Part model, mm, in its own coordinate system. Face numbers are marked on the shaded views. Round coordinates to 2 decimals unless told otherwise and drop trailing zeros. Loops run counter-clockwise (first coordinate to the right, second up) from the corner with the lowest first, then second, coordinate; pieces in that order, holes last.
1) Band-saw the part on D-D, the plane y = -23. Write the cut outline in (x, z), then the cut area to 3 significant figures.
2) Probe line 1 (Z direction, x = 17.5, y = 16); line 2 (Z direction, x = 5.5, y = 19.5); line 3 (Z direction, x = 2.5, y = 2). List the from-to ranges inside material, lowest first.
3) Band-saw the part on A-A, the plane y = 0. Write the cut outline in (x, z), then the cut area to 3 significant figures.
4) Band-saw the part on C-C, the plane x = -23. Write the cut outline in (y, z).
5) Band-saw the part on B-B, the plane z = 61.5. Write the cut outline in (x, y).
6) Drop flat-ended pins along their axis: P1, Ø8, axis at x = -9.5, y = 5, coming from the -Z side; P2, Ø9.5, axis at y = 38.5, z = -6.5, coming from the +X side; P3, Ø10, axis at y = -19, z = 82.5, coming from the +X side; P4, Ø7, axis at y = 26.5, z = -8.5, coming from the -X side. Give the stop position or say it passes through.
7) Mould opens along Z. For the marked faces 1, 2 and 3 say: +Z half, -Z half, draft (parallel to the pull), parting line (faces both ways), or undercut.
from build123d import *

# Parameters (mm, degrees)
SKETCH1_R                = 13.7
BOSS_EXTRUDE1_DEPTH      = 101
SKETCH5_W                = 55.5
SKETCH5_H                = 56.561345004
BOSS_EXTRUDE2_DEPTH      = 2.6
CUT_EXTRUDE4_DEPTH       = 2.6
BOSS_EXTRUDE4_DEPTH      = 6
SKETCH8_W                = 33.3
SKETCH8_H                = 11.7
BOSS_EXTRUDE5_DEPTH      = 2.8
SKETCH9_W                = 33.3
SKETCH9_H                = 2.7
BOSS_EXTRUDE6_DEPTH      = 22.2
FILLET2_R                = 5
REVOLVE1_ANGLE           = 40
REVOLVE1_OTHER_WAY_ANGLE = 40
FILLET4_R                = 6
FILLET5_R                = 6


with BuildPart() as part:
    # Sketch1 → Boss-Extrude1 (new body)
    with BuildSketch(Plane.XY):
        with Locations(Location((0, 0, 0), (0, 0, 180))):
            Circle(SKETCH1_R)
    extrude(amount=BOSS_EXTRUDE1_DEPTH)

    # Sketch5 → Boss-Extrude2 (add)
    with BuildSketch(Plane(origin=(0, 0, 0), x_dir=(-1, 0, 0), z_dir=(0, 0, -1))):
        Rectangle(SKETCH5_W, SKETCH5_H)
    extrude(amount=BOSS_EXTRUDE2_DEPTH)

    # Sketch6 → Cut-Extrude4 (cut)
    with BuildSketch(Plane(origin=(0, 0, -2.6), x_dir=(-1, 0, 0), z_dir=(0, 0, -1))):
        Polygon((27.75, 28.280672502), (18.35, 28.280672502), (27.75, 16.680672502), align=None)
        Polygon((-16.15, -28.280672502), (-27.75, -16.680672502), (-27.75, -28.280672502), align=None)
        Polygon((27.75, -18.880672502), (18.35, -28.280672502), (27.75, -28.280672502), align=None)
        Polygon((-27.75, 16.680672502), (-27.75, 28.280672502), (-16.15, 28.280672502), align=None)
    extrude(amount=-CUT_EXTRUDE4_DEPTH, mode=Mode.SUBTRACT)

    # Sketch7 → Boss-Extrude4 (add)
    with BuildSketch(Plane(origin=(0, 0, -2.6), x_dir=(-1, 0, 0), z_dir=(0, 0, -1))):
        Polygon((1.1, 25.680672502), (16.366645995, 25.680672502), (16.366645995, 22.680672502), (-16.933354005, 22.680672502), (-16.933354005, 25.680672502), align=None)
    extrude(amount=BOSS_EXTRUDE4_DEPTH)

    # Sketch8 → Boss-Extrude5 (add)
    with BuildSketch(Plane(origin=(0, 0, -8.6), x_dir=(-1, 0, 0), z_dir=(0, 0, -1))):
        with Locations((-0.283354005, 19.830672502)):
            Rectangle(SKETCH8_W, SKETCH8_H)
    extrude(amount=BOSS_EXTRUDE5_DEPTH)

    # Sketch9 → Boss-Extrude6 (add)
    with BuildSketch(Plane(origin=(0, 25.680672502, 0), x_dir=(1, 0, 0), z_dir=(0, 1, 0))):
        with Locations((0.283354005, 10.05)):
            Rectangle(SKETCH9_W, SKETCH9_H)
    extrude(amount=BOSS_EXTRUDE6_DEPTH)

    # Fillet2
    # the kernel refuses this fillet: 5 mm, written as the material it adds along each edge
    with BuildSketch(Plane(origin=(-16.366645995, 25.680672502, -2.6), x_dir=(0, 1, 0), z_dir=(1, 0, 0))) as fillet2_piece_1_section:
        with BuildLine():
            CenterArc((5, -4.38634244), FILLET2_R, 118.685402014, 61.314597986)
            Line((0, -4.38634244), (-0.1, -4.38634244))
            Line((-0.1, -4.38634244), (-0.1, 0))
            Line((-0.1, 0), (0, 0.1))
            ThreePointArc((0, 0.1), (1.3, 0.1), (2.552, 0.087726849))
            Line((2.552, 0.087726849), (2.6, 0))
        make_face()
    fillet2_piece_1 = extrude(amount=33.3, mode=Mode.PRIVATE)
    fillet2_piece_1 = split(fillet2_piece_1, bisect_by=Plane(origin=(9.175527955, 35.255144547, -3.690317045), z_dir=(-0.7071067811865442, -0.7071067811865509, 0)), keep=Keep.TOP, mode=Mode.PRIVATE)
    add(fillet2_piece_1)
    with BuildSketch(Plane(origin=(-16.366645995, 22.680672502, -2.6), x_dir=(0, -1, 0), z_dir=(1, 0, 0))) as fillet2_piece_2:
        with BuildLine():
            CenterArc((FILLET2_R, FILLET2_R), FILLET2_R, 180, 90)
            Line((0, FILLET2_R), (-FILLET2_R * 0.02, FILLET2_R))
            Line((-FILLET2_R * 0.02, FILLET2_R), (-FILLET2_R * 0.02, -FILLET2_R * 0.02))
            Line((-FILLET2_R * 0.02, -FILLET2_R * 0.02), (FILLET2_R, -FILLET2_R * 0.02))
            Line((FILLET2_R, -FILLET2_R * 0.02), (FILLET2_R, 0))
        make_face()
    extrude(amount=33.3)
    with BuildSketch(Plane(origin=(-16.366645995, 22.680672502, -8.6), x_dir=(0, -1, 0), z_dir=(1, 0, 0)), Plane(origin=(16.933354005, 25.680672502, -8.7), x_dir=(0, 1, 0), z_dir=(-1, 0, 0))) as fillet2_piece_3:
        with BuildLine():
            CenterArc((FILLET2_R, -FILLET2_R), FILLET2_R, 90, 90)
            Line((0, -FILLET2_R), (-FILLET2_R * 0.02, -FILLET2_R))
            Line((-FILLET2_R * 0.02, -FILLET2_R), (-FILLET2_R * 0.02, FILLET2_R * 0.02))
            Line((-FILLET2_R * 0.02, FILLET2_R * 0.02), (FILLET2_R, FILLET2_R * 0.02))
            Line((FILLET2_R, FILLET2_R * 0.02), (FILLET2_R, 0))
        make_face()
    extrude(amount=33.3)

    # Sketch10 → Revolve1 (revolve)
    with BuildSketch(Plane.ZY):
        with BuildLine():
            Line((101, 13.7), (101, 18.607528808))
            add(Edge.make_bspline(
                [(101, 18.607528808), (100.71882797, 21.282411004), (99.289162218, 18.607528808)],
                knots=[0, 0, 0, 1, 1, 1], degree=2))
            ThreePointArc((99.289162218, 18.607528808), (93.932259194, 15.08494276), (87.67231063, 13.7))
            Line((87.67231063, 13.7), (101, 13.7))
        make_face()
    revolve(axis=Axis((0, 0, 101.100764075), (0, 0, -1)), revolution_arc=REVOLVE1_ANGLE)

    # Sketch10 → Revolve1 other way (revolve)
    with BuildSketch(Plane.ZY):
        with BuildLine():
            Line((101, 13.7), (101, 18.607528808))
            add(Edge.make_bspline(
                [(101, 18.607528808), (100.71882797, 21.282411004), (99.289162218, 18.607528808)],
                knots=[0, 0, 0, 1, 1, 1], degree=2))
            ThreePointArc((99.289162218, 18.607528808), (93.932259194, 15.08494276), (87.67231063, 13.7))
            Line((87.67231063, 13.7), (101, 13.7))
        make_face()
    revolve(axis=Axis((0, 0, 101.100764075), (0, 0, 1)), revolution_arc=REVOLVE1_OTHER_WAY_ANGLE)

    # Fillet4
    fillet4_edges = [part.edges().sort_by_distance(p)[0] for p in [
        (8.806190253, 10.494808871, 94.336155315),
    ]]
    fillet(fillet4_edges, radius=FILLET4_R)

    # Fillet5
    fillet5_edges = [part.edges().sort_by_distance(p)[0] for p in [
        (-8.806190253, 10.494808871, 94.336155315),
    ]]
    fillet(fillet5_edges, radius=FILLET5_R)


solid = part.part
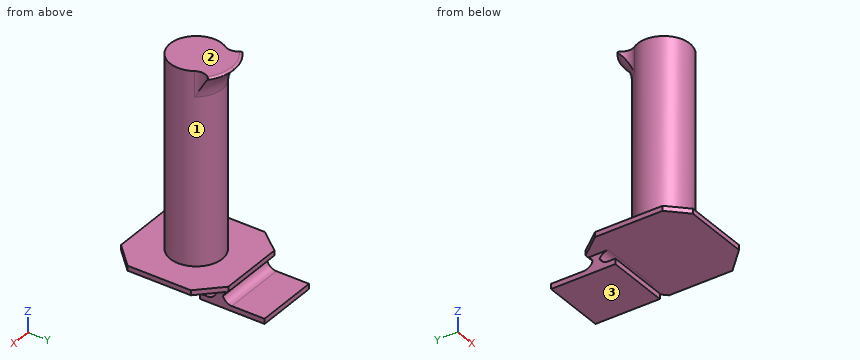
Reported:
1. outline: (-23.63, -2.6) - (21.43, -2.6) - (21.43, 0) - (-23.63, 0) - close
1. area: 117 mm2
2. line 1: z = -2.6 to 0
2. line 2: z = -11.4 to -8.26, -2.94 to 0
2. line 3: z = -2.6 to 101
3. outline: (-27.75, -2.6) - (27.75, -2.6) - (27.75, 0) - (13.7, 0) - (13.7, 101) - (-13.7, 101) - (-13.7, 0) - (-27.75, 0) - close
3. area: 2,910 mm2
4. outline: (-23.63, -2.6) - (22.54, -2.6) - (22.54, 0) - (-23.63, 0) - close
5. outline: circle Ø27.4 at (0, 0)
6. P1: stops at z = -2.6
6. P2: stops at x = 16.93
6. P3: passes through
6. P4: stops at x = -16.37
7. face 1: undercut
7. face 2: +Z half
7. face 3: -Z half
